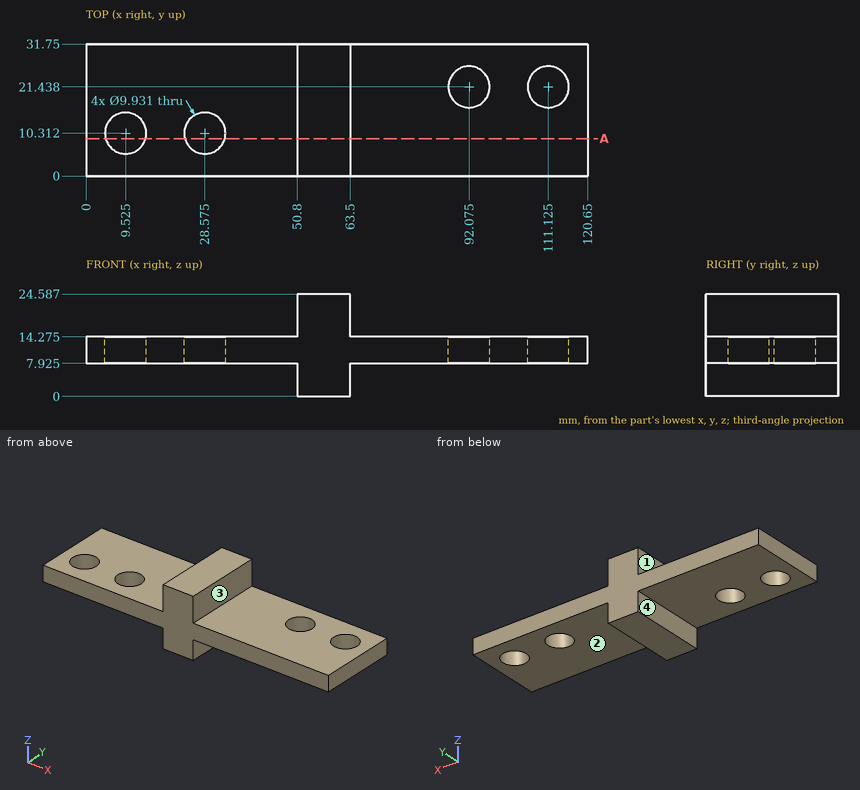
Check sheet for the drawn part. Datum: minimum x, y, z corner. Units: mm. A direction names the side the tool comes from. Give positions to 0.01 mm unless a question says otherwise; leave off trailing zeros.
1. Depth check by flat-ended pin: pin 1 (4 mm diameter, centred on y = 14.5, z = 4, fed in from +X); pin 2 (9.5 mm diameter, centred on x = 37.5, y = 16.5, fed in from -Z) (1 decimal); pin 3 (16 mm diameter, centred on x = 93, y = 11, fed in from +Z) (1 decimal). Enter the tip coordinate at first touch or a pass-through.
Completed:
pin 1: stops at x = 63.5
pin 2: stops at z = 7.9
pin 3: stops at z = 14.3
2. Access from +Z, -Z, +X, -X, +Y, -Y to the whole of each face (thin tool, end or side, straight path). Record for the marked faces 1, 2, 3 and 4.
Completed:
face 1: +Z, -X, +Y, -Y
face 2: -Z, +X, +Y, -Y
face 3: +Z, +X, +Y, -Y
face 4: -Z, -X, +Y, -Y
3. Sectioned sample at A-A (y = 9). State how many separate pieces and enclosed holes the cut face has, then the cut area to 3 significant figures.
Completed:
separate pieces: 3
enclosed holes: 0
area: 876 mm2
4. Scan lines: line 1 (X direction, y = 11.5, z = 11.5); line 2 (X direction, y = 3, z = 18.5); line 3 (Z direction, x = 107, y = 5) (1 decimal). Record each from-to range of solid material in increasing order.
Completed:
line 1: x = 0 to 4.7, 14.35 to 23.75, 33.4 to 120.65
line 2: x = 50.8 to 63.5
line 3: z = 7.9 to 14.3
